from build123d import *

# Parameters (mm, degrees)
SKETCH1_W           = 50.8
SKETCH1_H           = 25.4
SKETCH1_W_2         = 47.625
SKETCH1_H_2         = 22.225
BOSS_EXTRUDE1_DEPTH = 469.9
SKETCH4_R           = 4.826
CUT_EXTRUDE3_DEPTH  = 1.5875
SKETCH5_R           = 2.5527
CUT_EXTRUDE4_DEPTH  = 1.5875
SKETCH6_R           = 2.5527
CUT_EXTRUDE5_DEPTH  = 26.4
SKETCH7_R           = 2.5527
SKETCH7_R_2         = 2.4892
CUT_EXTRUDE6_DEPTH  = 51.8
SKETCH10_R          = 2.4892
CUT_EXTRUDE8_DEPTH  = 1.5875
CHAMFER1_SIZE       = 0.762


with BuildPart() as part:
    # Sketch1 → Boss-Extrude1 (new body, symmetric)
    with BuildSketch(Plane.XY):
        Rectangle(SKETCH1_W, SKETCH1_H)
        Rectangle(SKETCH1_W_2, SKETCH1_H_2, mode=Mode.SUBTRACT)
    extrude(amount=BOSS_EXTRUDE1_DEPTH, both=True)

    # Sketch4 → Cut-Extrude3 (cut)
    with BuildSketch(Plane(origin=(0, 12.7, 0), x_dir=(1, 0, 0), z_dir=(0, 1, 0))):
        with Locations((-12.7, -457.2)):
            Circle(SKETCH4_R)
        with Locations((0, -457.2)):
            Circle(SKETCH4_R)
        with Locations((12.7, -457.2)):
            Circle(SKETCH4_R)
    extrude(amount=-CUT_EXTRUDE3_DEPTH, mode=Mode.SUBTRACT)

    # Sketch5 → Cut-Extrude4 (cut)
    with BuildSketch(Plane.XZ.offset(12.7)):
        with Locations((12.7, 457.2)):
            Circle(SKETCH5_R)
        with Locations((0, 457.2)):
            Circle(SKETCH5_R)
        with Locations((-12.7, 457.2)):
            Circle(SKETCH5_R)
    extrude(amount=-CUT_EXTRUDE4_DEPTH, mode=Mode.SUBTRACT)

    # Sketch6 → Cut-Extrude5 (cut, through all)
    with BuildSketch(Plane.XZ.offset(12.7)):
        with Locations((12.7, -457.2)):
            Circle(SKETCH6_R)
        with Locations((0, -457.2)):
            Circle(SKETCH6_R)
        with Locations((-12.7, -457.2)):
            Circle(SKETCH6_R)
    extrude(amount=-CUT_EXTRUDE5_DEPTH, mode=Mode.SUBTRACT)

    # Sketch7 → Cut-Extrude6 (cut, through all)
    with BuildSketch(Plane(origin=(25.4, 0, 0), x_dir=(0, 0, -1), z_dir=(1, 0, 0))):
        with Locations((431.8, 0)):
            Circle(SKETCH7_R)
        with Locations((444.5, 0)):
            Circle(SKETCH7_R)
        with Locations((-444.5, 3.175)):
            Circle(SKETCH7_R_2)
        with Locations((-431.8, 3.175)):
            Circle(SKETCH7_R_2)
    extrude(amount=-CUT_EXTRUDE6_DEPTH, mode=Mode.SUBTRACT)

    # Sketch10 → Cut-Extrude8 (cut)
    with BuildSketch(Plane(origin=(0, 12.7, 0), x_dir=(1, 0, 0), z_dir=(0, 1, 0))):
        with Locations((-12.7, -419.1)):
            Circle(SKETCH10_R)
        with Locations((12.7, -419.1)):
            Circle(SKETCH10_R)
        with Locations((-12.7, -406.4)):
            Circle(SKETCH10_R)
        with Locations((12.7, -406.4)):
            Circle(SKETCH10_R)
        with Locations((-12.7, -393.7)):
            Circle(SKETCH10_R)
        with Locations((12.7, -393.7)):
            Circle(SKETCH10_R)
        with Locations((-12.7, -381)):
            Circle(SKETCH10_R)
        with Locations((12.7, -381)):
            Circle(SKETCH10_R)
        with Locations((-12.7, -368.3)):
            Circle(SKETCH10_R)
        with Locations((12.7, -368.3)):
            Circle(SKETCH10_R)
        with Locations((-12.7, -355.6)):
            Circle(SKETCH10_R)
        with Locations((12.7, -355.6)):
            Circle(SKETCH10_R)
        with Locations((-12.7, -342.9)):
            Circle(SKETCH10_R)
        with Locations((12.7, -342.9)):
            Circle(SKETCH10_R)
        with Locations((-12.7, -330.2)):
            Circle(SKETCH10_R)
        with Locations((12.7, -330.2)):
            Circle(SKETCH10_R)
        with Locations((-12.7, -6.35)):
            Circle(SKETCH10_R)
        with Locations((12.7, -6.35)):
            Circle(SKETCH10_R)
        with Locations((-12.7, 6.35)):
            Circle(SKETCH10_R)
        with Locations((12.7, 6.35)):
            Circle(SKETCH10_R)
        with Locations((-12.7, 19.05)):
            Circle(SKETCH10_R)
        with Locations((12.7, 19.05)):
            Circle(SKETCH10_R)
        with Locations((-12.7, 31.75)):
            Circle(SKETCH10_R)
        with Locations((12.7, 31.75)):
            Circle(SKETCH10_R)
        with Locations((-12.7, 44.45)):
            Circle(SKETCH10_R)
        with Locations((12.7, 44.45)):
            Circle(SKETCH10_R)
        with Locations((-12.7, 57.15)):
            Circle(SKETCH10_R)
        with Locations((12.7, 57.15)):
            Circle(SKETCH10_R)
        with Locations((-12.7, 69.85)):
            Circle(SKETCH10_R)
        with Locations((12.7, 69.85)):
            Circle(SKETCH10_R)
        with Locations((-12.7, 82.55)):
            Circle(SKETCH10_R)
        with Locations((12.7, 82.55)):
            Circle(SKETCH10_R)
        with Locations((-12.7, 95.25)):
            Circle(SKETCH10_R)
        with Locations((12.7, 95.25)):
            Circle(SKETCH10_R)
    extrude(amount=-CUT_EXTRUDE8_DEPTH, mode=Mode.SUBTRACT)

    # Chamfer1
    chamfer1_edges = [part.edges().sort_by_distance(p)[0] for p in [
        (0, 12.7, -469.9),
    ]]
    chamfer(chamfer1_edges, length=CHAMFER1_SIZE)


solid = part.part
Check sheet for the modelled part. Datum: model origin and axes. Units: mm. A direction names the side the tool comes from. Coordinates: 2 decimals unless noted, no trailing zeros. Loops run counter-clockwise (first coordinate to the right, second up) from the corner with the lowest first, then second, coordinate; pieces in that order, holes last. Notation, with made-up numbers: (45, 7.25) -> (92, 7.25) arc R18 cw to (92, 13.25) -> close; hole circle Ø10 at (-32.5, -3). An arc over 180 degrees is marked (long way). Answer in a Markdown table with one row per item.
1. Release check for a two-part mould opening along X. For faces 3 (the face through (23.812, 0, 7)), 4 (the face through (0, -11.112, 7)), 5 (the face through (-0.1, -11.3, -469.9)), 6 (the face through (25.4, 0, 7)) record: released by +X, released by -X, zero draft, split by the parting line, or undercut.
Check values:
| item | result |
|---|---|
| face 3 | undercut |
| face 4 | undercut |
| face 5 | zero draft |
| face 6 | released by +X |
2. Sectioned sample at A-A, the plane z = -177.5. Record the boundary of the cut face in (x, y).
Check values:
| item | result |
|---|---|
| outline | (-25.4, -12.7) -> (25.4, -12.7) -> (25.4, 12.7) -> (-25.4, 12.7) -> close; hole (-23.81, -11.11) -> (23.81, -11.11) -> (23.81, 11.11) -> (-23.81, 11.11) -> close |
3. Go/stop test with a flat-tipped pin: pin 1 (7.5 mm diameter, centred on x = -12.7, z = 457.2, fed in from +Y). Record where the tip stops, or that it passes through.
Check values:
| item | result |
|---|---|
| pin 1 | stops at y = -11.11 |
4. Access from +Z, -Z, +X, -X, +Y, -Y to the whole of each face (thin tool, end or side, straight path). Record for faces 1 (the face through (0, -12.7, 7)), 2 (the face through (0, 11.112, 7)).
Check values:
| item | result |
|---|---|
| face 1 | +Z, -Z, +X, -X, -Y |
| face 2 | +Z, -Z |
5. Material ranges on line 1 along X through (y, z) = (12.15, -6.35); line 2 along X through (y, z) = (-12.05, 457.2); line 3 along X through (y, z) = (11.8, 457.2), recorded low to high. Write a range as [from, to].
Check values:
| item | result |
|---|---|
| line 1 | x = [-25.4, -15.19], [-10.21, 10.21], [15.19, 25.4] |
| line 2 | x = [-25.4, -15.25], [-10.15, -2.55], [2.55, 10.15], [15.25, 25.4] |
| line 3 | x = [-25.4, -17.53], [-7.87, -4.83], [4.83, 7.87], [17.53, 25.4] |
